Geometry check sheet. Reference: the model listing, model coordinates, mm. Face numbers are marked on the shaded views. A direction names the side the tool comes from. Coordinates: 2 decimals unless noted, no trailing zeros. Order: outer loops, then holes, each group sorted by start corner. A loop starts at its lowest first (then second) coordinate and runs counter-clockwise, first axis right, second up. Notation, with made-up numbers: (86.5, 78.25) - (124.5, 78.25) arc R21 cw to (124.5, 108.25) - close; hole circle Ø10 at (30.25, 50). An arc over 180 degrees is marked (long way). Return JSON: item names as keys, results as strings. Group by question number.
Item 1: Gauge pin test, flat end, axial feed: pin 1 (12 mm diameter, centred on x = 42.5, y = 44, fed in from -Z). Record the tip position at first contact, or that the pin passes through.
Item 2: Section check C-C on y = 26. Enter the section's corners in (x, z).
Item 3: Scan lines: probe 1 along Y at (x, z) = (-50.8, 73.75); probe 2 along X at (y, z) = (57, 73); probe 3 along Y at (x, z) = (30, 58.5). Record each from-to range of solid material in increasing order.
Item 4: Draft check along X on the marked faces 1, 2, 3 and 4. Enter one of: pulls with the +X half, pulls with the -X half, needs draft (parallel to the pull), parting line crosses it, or undercut.
Item 5: Section check B-B on x = 30.5. Enter the section's corners in (y, z), then the cut area to 3 significant figures.
Item 6: Section check A-A on z = 13.5. Enter the section's corners in (x, y), then the cut area to 3 significant figures.
Item 7: Section check D-D on z = 74. Enter the section's corners in (x, y).
Item 8: Tool access check on the marked faces 5 and 6. Record the directions out of +Z, -Z, +X, -X, +Y, -Y that give a thin tool (end or side, any length) a straight path to the whole face; none if there is none.
from build123d import *

# Parameters (mm, degrees)
F0_R     = 1.524
F1_DEPTH = 81.28
F2_W     = 13.3946808136
F2_H     = 17.3983402467
F2_W_2   = 15.2697945094
F2_H_2   = 13.5166846132
F3_DEPTH = 64.8716
F5_DEPTH = 5.842


# Not quite as in the source:
# - ends of sketch curves that miss each other by under 0.0002 mm in the source are joined


with BuildPart() as f1:
    # F0 (on Top) → F1 (new body)
    with BuildSketch(Plane.XY):
        with BuildLine():
            Line((57.15, -57.15), (57.15, 57.15))
            ThreePointArc((57.15, 57.15), (55.2901280605, 61.6401280605), (50.8, 63.5))
            Line((50.8, 63.5), (-50.8, 63.5))
            ThreePointArc((-50.8, 63.5), (-55.2901280605, 61.6401280605), (-57.15, 57.15))
            Line((-57.15, 57.15), (-57.15, -57.15))
            ThreePointArc((-57.15, -57.15), (-55.2901280605, -61.6401280605), (-50.8, -63.5))
            Line((-50.8, -63.5), (50.8, -63.5))
            ThreePointArc((50.8, -63.5), (55.2901280605, -61.6401280605), (57.15, -57.15))
        make_face()
        with Locations((-50.8, -57.15)):
            Circle(F0_R, mode=Mode.SUBTRACT)
        with Locations((50.8, -57.15)):
            Circle(F0_R, mode=Mode.SUBTRACT)
        with Locations((-50.8, 57.15)):
            Circle(F0_R, mode=Mode.SUBTRACT)
        with BuildLine():
            Line((-43.2651408, 60.96), (43.2651408, 60.96))
            ThreePointArc((43.2651408, 60.96), (44.4892438959, 60.34382576), (44.7235034291, 58.993558544))
            ThreePointArc((44.7235034291, 58.993558544), (46.3098719395, 52.6598719395), (52.643558117, 51.0735048367))
            ThreePointArc((52.643558117, 51.0735048367), (53.99382576, 50.8392438959), (54.61, 49.6151408))
            Line((54.61, 49.6151408), (54.61, -49.6151408))
            ThreePointArc((54.61, -49.6151408), (53.99382576, -50.8392438959), (52.643558544, -51.0735034291))
            ThreePointArc((52.643558544, -51.0735034291), (46.3098719395, -52.6598719395), (44.7235048367, -58.993558117))
            ThreePointArc((44.7235048367, -58.993558117), (44.4892438959, -60.34382576), (43.2651408, -60.96))
            Line((43.2651408, -60.96), (-43.2651408, -60.96))
            ThreePointArc((-43.2651408, -60.96), (-44.4892438959, -60.34382576), (-44.7235034291, -58.993558544))
            ThreePointArc((-44.7235034291, -58.993558544), (-46.3098719395, -52.6598719395), (-52.643558117, -51.0735048367))
            ThreePointArc((-52.643558117, -51.0735048367), (-53.99382576, -50.8392438959), (-54.61, -49.6151408))
            Line((-54.61, -49.6151408), (-54.61, 49.6151408))
            ThreePointArc((-54.61, 49.6151408), (-53.99382576, 50.8392438959), (-52.643558544, 51.0735034291))
            ThreePointArc((-52.643558544, 51.0735034291), (-46.3098719395, 52.6598719395), (-44.7235048367, 58.993558117))
            ThreePointArc((-44.7235048367, 58.993558117), (-44.4892438959, 60.34382576), (-43.2651408, 60.96))
        make_face(mode=Mode.SUBTRACT)
        with Locations((50.8, 57.15)):
            Circle(F0_R, mode=Mode.SUBTRACT)
    extrude(amount=F1_DEPTH)

    # F2 (on face) → F3 (cut)
    with BuildSketch(Plane(origin=(0, 0, 0), x_dir=(1, 0, 0), z_dir=(0, 0, -1))):
        with Locations((47.9126595932, 52.2608298767)):
            Rectangle(F2_W, F2_H)
        Polygon((-54.61, 60.96), (-54.61, 45.5632209778), (-42.4256250262, 45.9913872182), (-42.4256250262, 60.96), align=None)
        Polygon((37.4062317246, -45.9566726098), (37.9334576428, -60.96), (54.61, -60.96), (54.61, -45.9566726098), align=None)
        with Locations((-46.9751027453, -54.2016576934)):
            Rectangle(F2_W_2, F2_H_2)
    extrude(amount=-F3_DEPTH, mode=Mode.SUBTRACT)

    # F4 (on Top) → F5 (join)
    with BuildSketch(Plane.XY):
        Polygon((-45.8822585642, -55.3943701088), (-55.0047931408, -55.3943701088), (-54.9012337958, -60.975112021), (-45.8822585642, -60.975112021), align=None)
        Polygon((-45.4961853886, 60.9891191125), (-54.7619216034, 60.9891191125), (-54.6583622584, 55.4083772004), (-45.4961853886, 55.4083772004), align=None)
        Polygon((54.7389825022, 60.9891191125), (45.6164479256, 60.9891191125), (45.7200072706, 55.4083772004), (54.7389825022, 55.4083772004), align=None)
        Polygon((54.6354231571, -55.3943701088), (45.5128885806, -55.3943701088), (45.6164479256, -60.975112021), (54.6354231571, -60.975112021), align=None)
    extrude(amount=F5_DEPTH)


solid = f1.part
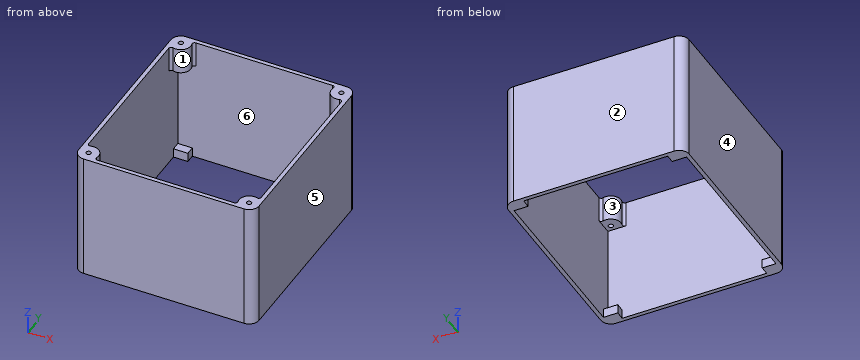
Computed:
{
 "1": {"pin 1": "passes through"},
 "2": {"outline": "(-57.15, 0) - (-54.61, 0) - (-54.61, 81.28) - (-57.15, 81.28) - close; (54.61, 0) - (57.15, 0) - (57.15, 81.28) - (54.61, 81.28) - close"},
 "3": {"probe 1": "y = -63.5 to -58.67, -55.63 to -50.8, 50.8 to 55.63, 58.67 to 63.5", "probe 2": "x = -57.15 to -52.32, -49.28 to -44.45, 44.45 to 49.28, 52.32 to 57.15", "probe 3": "y = -63.5 to -60.96, 60.96 to 63.5"},
 "4": {"face 1": "undercut", "face 2": "needs draft", "face 3": "undercut", "face 4": "pulls with the -X half"},
 "5": {"outline": "(-63.5, 0) - (-60.96, 0) - (-60.96, 81.28) - (-63.5, 81.28) - close; (60.96, 0) - (63.5, 0) - (63.5, 81.28) - (60.96, 81.28) - close", "area": "413 mm²"},
 "6": {"outline": "(-57.15, -57.15) arc R6.35 ccw to (-50.8, -63.5) - (50.8, -63.5) arc R6.35 ccw to (57.15, -57.15) - (57.15, 57.15) arc R6.35 ccw to (50.8, 63.5) - (-50.8, 63.5) arc R6.35 ccw to (-57.15, 57.15) - close; hole (-54.61, -60.96) - (54.61, -60.96) - (54.61, 60.96) - (-54.61, 60.96) - close", "area": "1,170 mm²"},
 "7": {"outline": "(-57.15, -57.15) arc R6.35 ccw to (-50.8, -63.5) - (50.8, -63.5) arc R6.35 ccw to (57.15, -57.15) - (57.15, 57.15) arc R6.35 ccw to (50.8, 63.5) - (-50.8, 63.5) arc R6.35 ccw to (-57.15, 57.15) - close; hole (-54.61, -49.62) arc R1.52 ccw to (-52.64, -51.07) arc R6.35 cw to (-44.72, -58.99) arc R1.52 ccw to (-43.27, -60.96) - (43.27, -60.96) arc R1.52 ccw to (44.72, -58.99) arc R6.35 cw to (52.64, -51.07) arc R1.52 ccw to (54.61, -49.62) - (54.61, 49.62) arc R1.52 ccw to (52.64, 51.07) arc R6.35 cw to (44.72, 58.99) arc R1.52 ccw to (43.27, 60.96) - (-43.27, 60.96) arc R1.52 ccw to (-44.72, 58.99) arc R6.35 cw to (-52.64, 51.07) arc R1.52 ccw to (-54.61, 49.62) - close; hole circle Ø3.05 at (-50.8, -57.15); hole circle Ø3.05 at (-50.8, 57.15); hole circle Ø3.05 at (50.8, -57.15); hole circle Ø3.05 at (50.8, 57.15)"},
 "8": {"face 5": "+Z, -Z, +X, +Y, -Y", "face 6": "none"}
}
